Read the model definition and answer for the solid it produces. Units are mm, in the model's axes. A direction names the side the tool comes from. Coordinates: 2 decimals unless noted, no trailing zeros. Write each loop counter-clockwise with the first axis right and the second up, starting at its lowest first coordinate (ties: lowest second). Pieces come first, ordered by that corner, then holes.
1) Which of the six approach directions +Z, -Z, +X, -X, +Y, -Y give full straight-line access (tool end or side, diameter ignored) to faces 4 (the face through (2.845, 0, 2)), 5 (the face through (47.295, 0, 0)), 6 (the face through (1, 0, -1.194))?
2) Find the intervals of material crossed by line 1 (X direction, y = 0.55, z = 0.2); line 2 (Y direction, x = 44, z = 0.15); line 3 (X direction, y = 0.9, z = -1.4), in increasing order.
3) The part is cut by section A-A (x = 27). Determine the outline of the cut face in (y, z).
4) Determine the mould class of faces 1 (the face through (0, -1, -1)), 2 (the face through (1.875, -0.041, -0.186)), 3 (the face through (25.3, -0.31, -1.39)) for opening direction Y: +Y half, -Y half, draft (parallel to the pull), parting line (faces both ways), or undercut.
from build123d import *

# Parameters (mm, degrees)
FILLET1_R   = 0.2286
HEX_2_DEPTH = 1.2954


with BuildPart() as part:
    # BodySke → Base-Revolve (revolve)
    with BuildSketch(Plane.XY):
        Polygon((0, 0), (0, 2.0447), (0.2794, 2.3241), (2.8448, 2.3241), (2.8448, 1.4224), (46.91634, 1.4224), (47.2948, 1.04394), (47.2948, 0), align=None)
    revolve(axis=Axis((-31.75, 0, 0), (1, 0, 0)))

    # Fillet1
    fillet1_edges = [part.edges().sort_by_distance(p)[0] for p in [
        (2.8448, -1.4224, 0),
    ]]
    fillet(fillet1_edges, radius=FILLET1_R)

    # Sketch2 → Hex-PreBroach (revolve, cut)
    with BuildSketch(Plane.XY):
        Polygon((0, 1.1938), (1.2954, 1.1938), (1.984640751, 0), (0, 0), align=None)
    revolve(axis=Axis((0, 0, 0), (1, 0, 0)), mode=Mode.SUBTRACT)

    # Sketch3 → Hex 2 (cut)
    with BuildSketch(Plane(origin=(0, 0, 0), x_dir=(0, 0.5, 0.866025404), z_dir=(-1, 0, 0))):
        Polygon((0.689240751, 1.1938), (-0.689240751, 1.1938), (-1.378481503, 0), (-0.689240751, -1.1938), (0.689240751, -1.1938), (1.378481503, 0), align=None)
    extrude(amount=-HEX_2_DEPTH, mode=Mode.SUBTRACT)


solid = part.part
Reported:
1. face 4: +X
1. face 5: +Z, -Z, +X, +Y, -Y
1. face 6: -X
2. line 1: x = 1.65 to 47.29
2. line 2: y = -1.41 to 1.41
2. line 3: x = 0 to 2.84
3. outline: circle Ø2.84 at (0, 0)
4. face 1: draft
4. face 2: undercut
4. face 3: parting line
